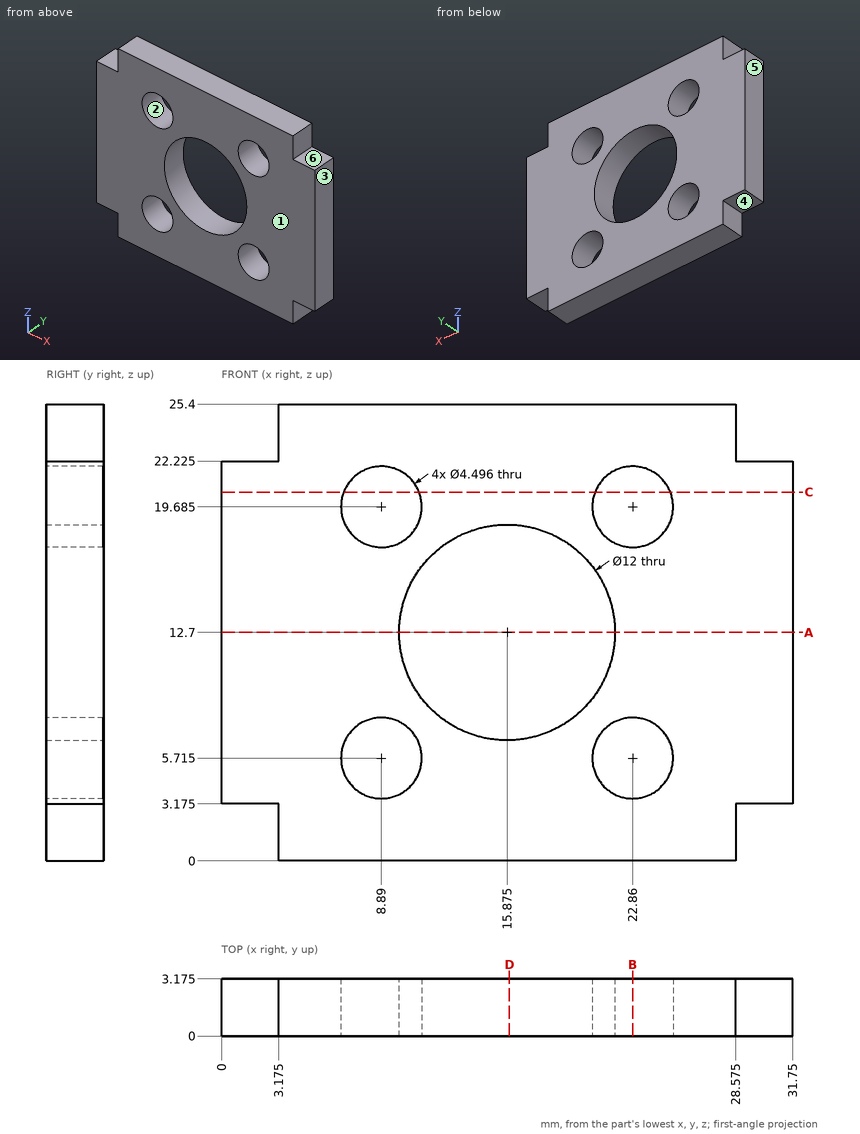
Verification items for this drawing (mm, ordinates from the low corner). A direction names the side the tool comes from. Coordinates: 2 decimals unless noted, no trailing zeros. Write each loop counter-clockwise with the first axis right and the second up, starting at its lowest first coordinate (ties: lowest second). Pieces come first, ordered by that corner, then holes. Notation, with made-up numbers: M 76,48 L 134,48 A21 ccw 134,68 Z; hole C 28.25,-11 d3. An arc over 180 degrees is marked long. Use CSV: the item, a comma, the result in double quotes.
Q1. Thickness scan on line 1 along Z through (x, y) = (22.86, 1.5); line 2 along X through (y, z) = (2, 21.25); line 3 along Z through (x, y) = (8.5, 2.8). Record the ranges inside material, lowest first. Write a range as [from, to].
Computed values:
line 1,"[0, 3.47], [7.96, 17.44], [21.93, 25.4]"
line 2,"[0, 7.28], [10.5, 21.25], [24.47, 31.75]"
line 3,"[0, 3.5], [7.93, 17.47], [21.9, 25.4]"
Q2. Set-up check for the marked faces 4, 5 and 6: record each of +Z, -Z, +X, -X, +Y, -Y from which the full face is reachable in a straight line by a thin tool's end or side.
Computed values:
face 4,"-Z, -X, +Y, -Y"
face 5,"+Z, -Z, -X, +Y, -Y"
face 6,"+Z, +X, +Y, -Y"
Q3. Section check C-C, the plane z = 20.5. Enter the section's corners in (x, y) (3 decimals).
Computed values:
outline,"M 0,0 L 6.795,0 L 6.795,3.175 L 0,3.175 Z; M 10.985,0 L 20.765,0 L 20.765,3.175 L 10.985,3.175 Z; M 24.955,0 L 31.75,0 L 31.75,3.175 L 24.955,3.175 Z"
Q4. Section check D-D, the plane x = 16. Enter the section's corners in (y, z) (1 decimal).
Computed values:
outline,"M 0,0 L 3.2,0 L 3.2,6.7 L 0,6.7 Z; M 0,18.7 L 3.2,18.7 L 3.2,25.4 L 0,25.4 Z"
Q5. Section check B-B, the plane x = 22.86. Enter the section's corners in (y, z) (1 decimal), and give its area (3 significant figures).
Computed values:
outline,"M 0,0 L 3.2,0 L 3.2,3.5 L 0,3.5 Z; M 0,8 L 3.2,8 L 3.2,17.4 L 0,17.4 Z; M 0,21.9 L 3.2,21.9 L 3.2,25.4 L 0,25.4 Z"
area,"52.1 mm²"
Q6. Mould release check, pull along X, two halves, no side actions. Record for the marked faces 1, 2 and 3: pulls with the +X half, pulls with the -X half, needs draft (parallel to the pull), parting line crosses it, or undercut.
Computed values:
face 1,"needs draft"
face 2,"undercut"
face 3,"pulls with the +X half"
Q7. Section check A-A, the plane z = 12.7. Enter the section's corners in (x, y) (3 decimals), and give its area (3 significant figures).
Computed values:
outline,"M 0,0 L 9.875,0 L 9.875,3.175 L 0,3.175 Z; M 21.875,0 L 31.75,0 L 31.75,3.175 L 21.875,3.175 Z"
area,"62.7 mm²"
Q8. Go/stop test with flat-tipped pins: P1, Ø2.5, axis at x = 22.86, z = 19.685, coming from the +Y side; P2, Ø1, axis at x = 30.5, y = 1, coming from the +Z side (3 decimals). Record where each tip stops, or that it passes through.
Computed values:
P1,"through"
P2,"z = 22.225"
